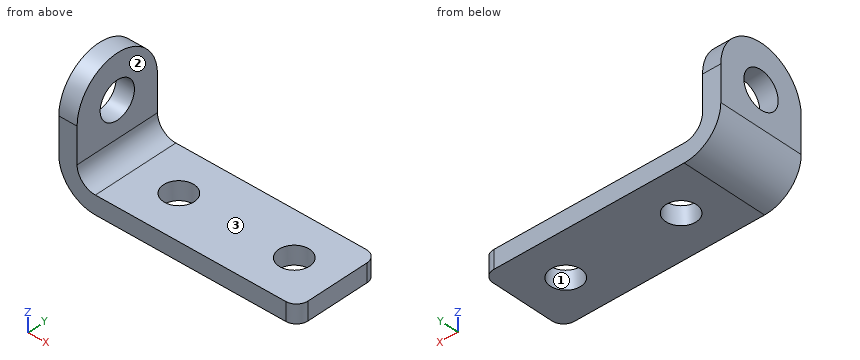
Autodesk Inventor part; units mm, degrees
ref_plane "YZ Plane" through (0, 0, 0) normal (1, 0, 0) x (0, 1, 0)
ref_plane "XZ Plane" through (0, 0, 0) normal (0, 1, 0) x (-1, 0, 0)
ref_plane "XY Plane" through (0, 0, 0) normal (0, 0, 1) x (1, 0, 0)
sketch "Sketch1" plane through (0, 0, 0) normal (0, 0, 1) x (1, 0, 0)
  line L0 (17.5, -7.5) -> (-17.5, -7.5)
  line L1 (-17.5, -7.5) -> (-17.5, 7.5)
  line L2 (-17.5, 7.5) -> (17.5, 7.5)
  line L3 (17.5, 7.5) -> (17.5, -7.5)
  line L4 (17.5, -7.5) -> (-17.5, 7.5) construction
  line L5 (-17.5, -7.5) -> (17.5, 7.5) construction
  line L6 (-10, 0) -> (10, 0) construction
  point P0 (0, 0)
  dimension "d0" = 35
  dimension "d1" = 15
  dimension "d2" = 20
  dimension "d3" = 7.5
extrude "Plate1" add sketch "Sketch1" along normal blind 3.175
sketch "Sketch2" plane through (-20.675, -7.5, 6.35) normal (-1, 0, 0) x (0, -1, 0)
  line L0 (-15, 0) -> (0, 0)
  line L1 (0, 0) -> (0, 13.65)
  line L2 (0, 13.65) -> (-15, 13.65)
  line L3 (-15, 13.65) -> (-15, 0)
edge flange "Flange1" height 20 angle 90 thickness 3.175 bend radius 3.175 thickness toward (-1, 0, 0) relief tear relief width 3.175 relief depth 1.5875 edges at (-17.5, 0, 3.175) wall of the first edge with corners at (-20.675, 7.5, 6.35) (-20.675, -7.5, 6.35) (-20.675, -7.5, 20) (-20.675, 7.5, 20)
bend "Bend1"
corner "Corner1"
hole "Hole1" at (-10, 0, 0) at (10, 0, 0) direction (0, 0, 1) diameter 5.3 end through all
sketch "Sketch3" plane through (-20.675, -7.5, 20) normal (1, 0, 0) x (0, 0, -1)
  line L0 (13.65, 0) -> (13.65, 15)
  line L1 (0, 15) -> (13.65, 15)
  line L2 (0, 15) -> (0, 0)
  line L3 (0, 0) -> (13.65, 0)
  circle A0 centre (7.5, 7.5) radius 7.5
  point P0 (20, 7.5)
  point P1 (0, 7.5)
  point P2 (7.5, 15)
  point P3 (7.5, 0)
hole "Hole2" at (-20.675, 0, 12.5) direction (-1, 0, 0) diameter 6.4 end through all
extrude "Extrusion1" cut sketch "Sketch3" against normal through all contours L3 L2 A0 | L2 L1 A0
fillet "Fillet1" radius 2 2 edges at (17.5, 7.5, 1.5875) (17.5, -7.5, 1.5875)
equation "\"d0\" = d2 + d1"
equation "\"d3\" = 0.5 * d1"
equation "\"d20\" = Thickness"
equation "\"d4\" = Thickness"
equation "\"d5\" = BendReliefWidth"
equation "\"d6\" = BendReliefDepth"
equation "\"d7\" = MinimumRemnant"
equation "\"d8\" = TransitionRadius"
equation "\"d11\" = BendRadius"
equation "\"d12\" = CornerReliefSize"
equation "\"d13\" = GapSize"
equation "\"d14\" = JacobiRadiusSize"
equation "\"BendReliefWidth\" = Thickness"
equation "\"BendReliefDepth\" = 0.5 * Thickness"
equation "\"CornerReliefSize\" = 4 * Thickness"
equation "\"MinimumRemnant\" = 2 * Thickness"
equation "\"TransitionRadius\" = BendRadius"
equation "\"JacobiRadiusSize\" = BendRadius"
equation "\"GapSize\" = Thickness"
properties part number "Inductive Sensor Bracket" material "Aluminum 6061"
Input: part model. Units: mm. Frame: model coordinates. Face numbers are marked on the shaded views. Round coordinates to 2 decimals unless told otherwise and drop trailing zeros. Loops run counter-clockwise (first coordinate to the right, second up) from the corner with the lowest first, then second, coordinate; pieces in that order, holes last. Notation, with made-up numbers: (-11.5, 67.25) -> (17.5, 67.25) arc R33 ccw to (17.5, 99.25) -> close; hole circle Ø5 at (39.25, 89.5). An arc over 180 degrees is marked (long way). One line per item, written item: value.
(1) Section A-A (x = 10). Return the cut outline in (y, z) (3 decimals).
Geometry check:
outline: (-7.5, 0) -> (-2.65, 0) -> (-2.65, 3.175) -> (-7.5, 3.175) -> close; (2.65, 0) -> (7.5, 0) -> (7.5, 3.175) -> (2.65, 3.175) -> close
(2) Material intervals for line 1 (Y direction, x = -10, z = 1.4); line 2 (X direction, y = 0, z = 0.75); line 3 (X direction, y = 0, z = 2.15), sorted ascending. Write a range as [from, to].
Geometry check:
line 1: [-7.5, -2.65], [2.65, 7.5]
line 2: [-20.49, -12.65], [-7.35, 7.35], [12.65, 17.5]
line 3: [-22.26, -12.65], [-7.35, 7.35], [12.65, 17.5]
(3) Section B-B (y = 0). Return the cut outline in (x, z) (3 decimals), plus the area to 3 significant figures.
Geometry check:
outline: (-23.85, 6.35) arc R6.35 ccw to (-17.5, 0) -> (-12.65, 0) -> (-12.65, 3.175) -> (-17.5, 3.175) arc R3.175 cw to (-20.675, 6.35) -> (-20.675, 9.3) -> (-23.85, 9.3) -> close; (-23.85, 15.7) -> (-20.675, 15.7) -> (-20.675, 20) -> (-23.85, 20) -> close; (-7.35, 0) -> (7.35, 0) -> (7.35, 3.175) -> (-7.35, 3.175) -> close; (12.65, 0) -> (17.5, 0) -> (17.5, 3.175) -> (12.65, 3.175) -> close
area: 124 mm2
(4) Section C-C (z = 14.5). Return the cut outline in (x, y) (3 decimals), plus the area to 3 significant figures.
Geometry check:
outline: (-23.85, -7.228) -> (-20.675, -7.228) -> (-20.675, -2.498) -> (-23.85, -2.498) -> close; (-23.85, 2.498) -> (-20.675, 2.498) -> (-20.675, 7.228) -> (-23.85, 7.228) -> close
area: 30.0 mm2
(5) Section D-D (z = 2.5). Return the cut outline in (x, y).
Geometry check:
outline: (-22.55, -7.5) -> (15.5, -7.5) arc R2 ccw to (17.5, -5.5) -> (17.5, 5.5) arc R2 ccw to (15.5, 7.5) -> (-22.55, 7.5) -> close; hole circle Ø5.3 at (-10, 0); hole circle Ø5.3 at (10, 0)
(6) Pin query (flat end, axial travel): pin 1 (6 mm diameter, centred on x = 10, y = 0, fed in from -Z); pin 2 (5 mm diameter, centred on y = 0, z = 15.5, fed in from +X) (3 decimals); pin 3 (6 mm diameter, centred on x = -9, y = -3.5, fed in from +Z) (3 decimals); pin 4 (1.5 mm diameter, centred on x = -19, y = -2, fed in from +Z). Return the tip coordinate at first contact, or that it passes through.
Geometry check:
pin 1: z = 0
pin 2: x = -20.675
pin 3: z = 3.175
pin 4: z = 4.11
(7) Mould query, pull axis X, two halves, no side actions, for the marked faces 1, 2 and 3. Classes: pulls with the +X half, pulls with the -X half, needs draft (parallel to the pull), parting line crosses it, or undercut.
Geometry check:
face 1: undercut
face 2: pulls with the +X half
face 3: needs draft
